```python
from build123d import *

# Parameters (mm, degrees)
F1_DEPTH  = 45
F3_W      = 4
F3_H      = 4.3
F4_DEPTH  = 16
F6_D      = 4.5
F6_DEPTH  = 30
F6_TIP    = 1.3519363928
F8_R      = 4
F11_W     = 8
F11_H     = 4.3
F12_DEPTH = 0.9
F13_W     = 8
F13_H     = 4.3
F14_DEPTH = 0.9
F15_R     = 2.99999
F2_R      = 1.95
F2_R_2    = 0.75
F16_DEPTH = 4.3


# Not quite as in the source:
# - a fillet or chamfer is up to 0.001 mm smaller than in the source, because OpenCascade refuses the exact size


with BuildPart() as f1:
    # F0 (on Front) → F1 (new body)
    with BuildSketch(Plane.XZ):
        Polygon((0, 0), (0, 4.3), (16, 4.3), (16, 0), (19, 0), (19, 7.3), (-3, 7.3), (-3, 0), align=None)
    extrude(amount=F1_DEPTH)

    # F3 (on face) → F4 (join)
    with BuildSketch(Plane.YZ):
        with Locations((-2, 2.15)):
            Rectangle(F3_W, F3_H)
    extrude(amount=F4_DEPTH)

    # F6
    with Locations(Plane(origin=(0, 0, 0), x_dir=(-1, 0, 0), z_dir=(0, 1, 0))):
        with Locations((-8, 0)):
            Hole(F6_D / 2, depth=F6_DEPTH)
            with Locations((0, 0, -(F6_DEPTH + F6_TIP / 2))):  # 118° drill point
                Cone(0, F6_D / 2, F6_TIP, mode=Mode.SUBTRACT)


with BuildPart() as f7_1:
    # F7: copy of F1
    add(f1.part.moved(Location((31.9, 0.1, 0))))


with BuildPart() as f1_1:
    add(f1.part)

    # F8
    f8_edges = [f1_1.edges().sort_by_distance(p)[0] for p in [
        (-3, -22.5, 7.3),
        (19, -22.5, 7.3),
    ]]
    fillet(f8_edges, radius=F8_R)


with BuildPart() as f10_1:
    # F10: copy of F1
    add(f1_1.part.moved(Location((35.6, 1.7, 0))))


with BuildPart() as f1_2:
    add(f1_1.part)

    # F11 (on face) → F12 (join)
    with BuildSketch(Plane.YZ):
        with Locations((-41, 2.15)):
            Rectangle(F11_W, F11_H)
    extrude(amount=F12_DEPTH)

    # F13 (on face) → F14 (join)
    with BuildSketch(Plane(origin=(16, 0, 0), x_dir=(0, -1, 0), z_dir=(-1, 0, 0))):
        with Locations((41, 2.15)):
            Rectangle(F13_W, F13_H)
    extrude(amount=F14_DEPTH)

    # F15 (radius 3 in the source; OpenCascade refuses exactly that, so slightly less here)
    f15_edges = [f1_2.edges().sort_by_distance(p)[0] for p in [
        (8, -45, 7.3),
        (8, 0, 7.3),
    ]]
    fillet(f15_edges, radius=F15_R)

    # F2 (on face) → F16 (join)
    with BuildSketch(Plane(origin=(0, 0, 4.3), x_dir=(1, 0, 0), z_dir=(0, 0, -1))):
        with Locations((2, 30)):
            Circle(F2_R)
        with Locations((2, 30)):
            Circle(F2_R_2, mode=Mode.SUBTRACT)
        with Locations((14, 30)):
            Circle(F2_R)
        with Locations((14, 30)):
            Circle(F2_R_2, mode=Mode.SUBTRACT)
        with Locations((2, 8)):
            Circle(F2_R)
        with Locations((2, 8)):
            Circle(F2_R_2, mode=Mode.SUBTRACT)
        with Locations((14, 8)):
            Circle(F2_R)
        with Locations((14, 8)):
            Circle(F2_R_2, mode=Mode.SUBTRACT)
    extrude(amount=F16_DEPTH)


solid = f1_2.part
```
The listing builds one solid part. Answer for the finished solid, in the listing's coordinates (mm). A direction names the side the tool comes from. Round coordinates to 2 decimals unless told otherwise and drop trailing zeros. Order: outer loops, then holes, each group sorted by start corner. A loop starts at its lowest first (then second) coordinate and runs counter-clockwise, first axis right, second up. Notation, with made-up numbers: (-35, -16) -> (-24, -16) arc R17 ccw to (-24, 7) -> close; hole circle Ø1 at (-9.75, 17.5). An arc over 180 degrees is marked (long way). Answer as CSV lines item,"result". Start each with the question number.
(1) The part is cut by section A-A (z = 2.75). Count the separate pieces of the cut face and the enclosed holes in it, then the cut area to 3 significant figures.
(2) For a pull along Y with two mould halves and no side action, classify faces 4 (the face through (12.563, -31.318, 2.18)), 5 (the face through (8, -22, 7.3)), 6 (the face through (7.9, -0.86, 6.4)), 7 (the face through (7.9, -44.14, 6.4)) as +Y half, -Y half, draft (parallel to the pull), parting line (faces both ways), or undercut.
(3) Find the intervals of material crossed by probe 1 along Y at (x, z) = (14, 1.2); probe 2 along X at (y, z) = (-32.5, 1.5); probe 3 along Y at (x, z) = (14.5, 2.5), in increasing order. Write a range as from..to.
(4) The part is cut by section B-B (y = -41). Determine the outline of the cut face in (x, z).
(5) A tool of negligible diameter and unlimited length cuts with its end or side. For faces 1 (the face through (0.4, -37, 2.1)), 2 (the face through (15.6, -45, 2.1)), 3 (the face through (15.1, -41, 2)), from which of +Z, -Z, +X, -X, +Y, -Y can it reach the whole face along a straight path? Write none if from no direction.
(6) The part is cut by section D-D (y = -8). Determine the outline of the cut face in (x, z), then the cut area to 3 significant figures.
(7) Flat-ended cylindrical pins translate along their axes: pin 1 Ø1.3 at (x, z) = (11, 3) entering from -Y; pin 2 Ø1.2 at (x, y) = (2, -30) entering from -Z. Find the tip coordinate at first contact, or state that the pin passes through.
Evaluation:
1,separate pieces,"5"
1,enclosed holes,"4"
1,area,"381 mm²"
2,face 4,"undercut"
2,face 5,"draft"
2,face 6,"+Y half"
2,face 7,"-Y half"
3,probe 1,"-31.95..-30.75, -29.25..-28.05, -9.95..-8.75, -7.25..-6.05, -4..0"
3,probe 2,"-3..0, 16..19"
3,probe 3,"-31.88..-30.56, -29.44..-28.12, -9.88..-8.56, -7.44..-6.12, -4..0"
4,outline,"(-3, 0) -> (0.9, 0) -> (0.9, 4.3) -> (15.1, 4.3) -> (15.1, 0) -> (19, 0) -> (19, 3.3) arc R4 ccw to (15, 7.3) -> (1, 7.3) arc R4 ccw to (-3, 3.3) -> close"
5,face 1,"-Z"
5,face 2,"+Z, -Z, +X, -X, -Y"
5,face 3,"-Z, -Y"
6,outline,"(-3, 0) -> (0, 0) -> (0, 4.3) -> (0.05, 4.3) -> (0.05, 0) -> (1.25, 0) -> (1.25, 4.3) -> (2.75, 4.3) -> (2.75, 0) -> (3.95, 0) -> (3.95, 4.3) -> (12.05, 4.3) -> (12.05, 0) -> (13.25, 0) -> (13.25, 4.3) -> (14.75, 4.3) -> (14.75, 0) -> (15.95, 0) -> (15.95, 4.3) -> (16, 4.3) -> (16, 0) -> (19, 0) -> (19, 3.3) arc R4 ccw to (15, 7.3) -> (1, 7.3) arc R4 ccw to (-3, 3.3) -> close"
6,area,"106 mm²"
7,pin 1,"y = -4"
7,pin 2,"z = 4.3"
